```python
from build123d import *

# Parameters (mm, degrees)
F0_R         = 10
F1_DEPTH     = 15
F2_R         = 15
F3_T1_DEPTH  = 32.0168478214
F3_T3_DEPTH  = 19.855092474
F3_T5_DEPTH  = 60.8257569496
F3_T7_DEPTH  = 65
F3_T9_DEPTH  = 54.2875458035
F3_T11_DEPTH = 15
F5_R         = 12
F6_DEPTH     = 12
F7_R         = 11.99999
F8_R         = 4.05
F9_DEPTH     = 27.001


# Not quite as in the source:
# - a fillet or chamfer that OpenCascade refuses, or shapes differently, is made with other operations: its cross-section is extruded or revolved along the edge and cut away or added
# - a fillet or chamfer is up to 0.001 mm smaller than in the source, because OpenCascade refuses the exact size


with BuildPart() as f1:
    # F0 (on Front) → F1 (new body)
    with BuildSketch(Plane.XZ):
        Polygon((-138.9475274131, 122.1416580278), (0, 0), (17.5, -71.8808303125), (45.5, -71.8808303125), (45.5, -56.8808303125), (39.5, -56.8808303125), (35, -62), (27, -62), (27, -12), (35, -12), (35, -20), (41, -20), (41, 0), (0, 53.2575148171), (-112.5385202719, 152.1843666577), align=None)
        with Locations((-67.1597420143, 85.6654484175)):
            Circle(F0_R, mode=Mode.SUBTRACT)
        with Locations((-89.6917734867, 105.4722037734)):
            Circle(F0_R, mode=Mode.SUBTRACT)
        with Locations((-44.6277105419, 65.8586930616)):
            Circle(F0_R, mode=Mode.SUBTRACT)
        with Locations((-22.0956790695, 46.0519377058)):
            Circle(F0_R, mode=Mode.SUBTRACT)
    extrude(amount=F1_DEPTH)

    # F2
    f2_edges = [f1.edges().sort_by_distance(p)[0] for p in [
        (-112.53852, -7.5, 152.184367),
        (-138.947527, -7.5, 122.141658),
    ]]
    fillet(f2_edges, radius=F2_R)

    # F3: fillet of radius 10 on 6 edges, made by hand

    # F3_s2 → F3_t1 (cut)
    with BuildSketch(Plane.XZ.offset(-8.5084239107)):
        with BuildLine():
            ThreePointArc((38.9238894384, 2.6967924145), (40.4667548395, -0.1814830349), (41, -3.4033695643))
            Line((41, -3.4033695643), (41.2, -3.4033695643))
            Line((41.2, -3.4033695643), (41.2, 0.0680673913))
            Line((41.2, 0.0680673913), (39.0823672272, 2.8187956541))
            Line((39.0823672272, 2.8187956541), (38.9238894384, 2.6967924145))
        make_face()
    extrude(amount=F3_T1_DEPTH, mode=Mode.SUBTRACT)

    # F3_s4 → F3_t3 (cut)
    with BuildSketch(Plane.XZ.offset(-2.427546237)):
        with BuildLine():
            ThreePointArc((-0.7293006428, 53.8986056762), (-0.0343212423, 53.2253561798), (0.5923370103, 52.4880904975))
            Line((0.5923370103, 52.4880904975), (0.750814799, 52.6100937371))
            Line((0.750814799, 52.6100937371), (0.1466310486, 53.3949065431))
            Line((0.1466310486, 53.3949065431), (-0.5972556071, 54.0488192193))
            Line((-0.5972556071, 54.0488192193), (-0.7293006428, 53.8986056762))
        make_face()
    extrude(amount=F3_T3_DEPTH, mode=Mode.SUBTRACT)

    # F3_s6 → F3_t5 (cut)
    with BuildSketch(Plane.XZ.offset(-22.9128784748)):
        with BuildLine():
            ThreePointArc((45.5, -66.0459817024), (43.8666002653, -60.5687561273), (39.5, -56.8808303125))
            Line((39.5, -56.8808303125), (39.58, -56.6975272847))
            ThreePointArc((39.58, -56.6975272847), (42.5, -56.6808303125), (45.5, -56.6808303125))
            Line((45.5, -56.6808303125), (45.7, -56.8808303125))
            Line((45.7, -56.8808303125), (45.7, -66.0459817024))
            Line((45.7, -66.0459817024), (45.5, -66.0459817024))
        make_face()
    extrude(amount=F3_T5_DEPTH, mode=Mode.SUBTRACT)

    # F3_s8 → F3_t7 (cut)
    with BuildSketch(Plane.XZ.offset(-25)):
        with BuildLine():
            ThreePointArc((35.5, -71.8808303125), (42.5710678119, -68.9518981244), (45.5, -61.8808303125))
            Line((45.5, -61.8808303125), (45.7, -61.8808303125))
            Line((45.7, -61.8808303125), (45.7, -72.0808303125))
            Line((45.7, -72.0808303125), (35.5, -72.0808303125))
            Line((35.5, -72.0808303125), (35.5, -71.8808303125))
        make_face()
    extrude(amount=F3_T7_DEPTH, mode=Mode.SUBTRACT)

    # F3_s10 → F3_t9 (cut)
    with BuildSketch(Plane.XZ.offset(-19.6437729018)):
        with BuildLine():
            ThreePointArc((15.6413136753, -64.2463208091), (19.1791155574, -69.7438737743), (25.3575091607, -71.8808303125))
            Line((25.3575091607, -71.8808303125), (25.3575091607, -72.0808303125))
            Line((25.3575091607, -72.0808303125), (17.3428498168, -72.0808303125))
            Line((17.3428498168, -72.0808303125), (15.4469897656, -64.2936306191))
            Line((15.4469897656, -64.2936306191), (15.6413136753, -64.2463208091))
        make_face()
    extrude(amount=F3_T9_DEPTH, mode=Mode.SUBTRACT)

    # F3_s12 → F3_t11 (join)
    with BuildSketch(Plane.XZ):
        with BuildLine():
            ThreePointArc((-2.3681074114, 2.0816819918), (-0.4151755765, -0.2512704506), (0.7458362887, -3.0635046691))
            Line((0.7458362887, -3.0635046691), (0.9401601984, -3.0161948591))
            Line((0.9401601984, -3.0161948591), (0.1794071839, 0.1085799033))
            Line((0.1794071839, 0.1085799033), (-2.2360623757, 2.2318955349))
            Line((-2.2360623757, 2.2318955349), (-2.3681074114, 2.0816819918))
        make_face()
    extrude(amount=F3_T11_DEPTH)

    # F5 (on face) → F6 (join)
    with BuildSketch(Plane(origin=(0, 0, 0), x_dir=(-1, 0, 0), z_dir=(0, 1, 0))):
        with Locations((111.3978201201, 124.552878143)):
            Circle(F5_R)
    extrude(amount=F6_DEPTH)

    # F7 (radius 12 in the source; OpenCascade refuses exactly that, so slightly less here)
    f7_edges = [f1.edges().sort_by_distance(p)[0] for p in [
        (-99.39782, 12, 124.552878),
    ]]
    fillet(f7_edges, radius=F7_R)

    # F8 (on face) → F9 (cut, through all)
    with BuildSketch(Plane.XZ.offset(15)):
        with Locations((-111.3978201201, 124.552878143)):
            Circle(F8_R)
    extrude(amount=-F9_DEPTH, mode=Mode.SUBTRACT)


solid = f1.part
```
Could you check a few things on this model? Use its own coordinates, in mm. A direction names the side the tool comes from. Round coordinates to 2 decimals unless told otherwise and drop trailing zeros. Loops run counter-clockwise (first coordinate to the right, second up) from the corner with the lowest first, then second, coordinate; pieces in that order, holes last. Notation, with made-up numbers: (44.5, 17.5) - (71.5, 17.5) arc R30 cw to (71.5, 52.5) - close; hole circle Ø9 at (-34, -18). An arc over 180 degrees is marked (long way). Answer in a Markdown table with one row per item. Add a question column.
(1) If we section it at A-A (x = -83): Please give me the cut outline in (y, z).
(2) If we section it at C-C (y = -9): Please give me the cut outline in (x, z).
(3) For faces 1 (the face through (41, -7, -12)), 2 (the face through (-65.9, -7.4, 57.93)), 3 (the face through (38, -7, -20)), 4 (the face through (37.282, -7.395, -59.405)), which set-ups out of +Z, -Z, +X, -X, +Y, -Y let a thin tool reach every point of the face, with its end or its side?
(4) I'm going to push flat-ended pins straight in: pin 1 (2 mm diameter, centred on y = -4, z = 84, fed in from -X); pin 2 (7.5 mm diameter, centred on y = -8, z = -36.5, fed in from +X); pin 3 (1 mm diameter, centred on y = 0, z = 54.5, fed in from -X); pin 4 (5 mm diameter, centred on x = 37.5, y = -6.5, fed in from -Z). Where does each tip first touch, or does it pass through?
(5) If we section it at D-D (x = 22.5): Please give me the cut outline in (y, z).
(6) I need wall thicknesses on line 1 along Z through (x, y) = (-92, -9.5); line 2 along Z through (x, y) = (-113, 5.75); line 3 along X through (y, z) = (-11.25, 61). Which ranges of each line are inside material? Lowest first, please.
(7) If we mould it in two halves opening along Z, with no side actions, what happens to faces 5 (the face through (31, -7, -12)), 6 (the face through (-125.697, -7.395, 137.216)), 7 (the face through (-38, -15, 54))? For each: pulls with the +Z half, pulls with the -Z half, needs draft (parallel to the pull), parting line crosses it, or undercut.
(8) If we section it at B-B (z = 62.5): Please give me the cut outline in (x, y), plus the area to 3 significant figures.
Model answer:
| question | item | result |
|---|---|---|
| 1 | outline | (-15, 72.96) - (0, 72.96) - (0, 98.04) - (-15, 98.04) - close; (-15, 112.9) - (0, 112.9) - (0, 126.22) - (-15, 126.22) - close |
| 2 | outline | (-129.04, 133.41) arc R15 ccw to (-127.68, 112.24) - (-2.37, 2.08) arc R10 cw to (0.75, -3.06) - (15.64, -64.25) arc R10 ccw to (25.36, -71.88) - (35.5, -71.88) arc R10 ccw to (45.28, -63.96) arc R10 ccw to (39.5, -56.88) - (35, -62) - (27, -62) - (27, -12) - (35, -12) - (35, -20) - (41, -20) - (41, -3.4) arc R10 ccw to (38.92, 2.7) - (0.59, 52.49) arc R10 ccw to (-0.73, 53.9) - (-101.27, 142.28) arc R15 ccw to (-122.44, 140.92) - close; hole circle Ø8.1 at (-111.4, 124.55); hole circle Ø20 at (-89.69, 105.47); hole circle Ø20 at (-67.16, 85.67); hole circle Ø20 at (-44.63, 65.86); hole circle Ø20 at (-22.1, 46.05) |
| 3 | face 1 | +Z, +X, +Y, -Y |
| 3 | face 2 | -Z, -X, +Y, -Y |
| 3 | face 3 | +X, +Y, -Y |
| 3 | face 4 | +Y, -Y |
| 4 | pin 1 | stops at x = -96.7 |
| 4 | pin 2 | stops at x = 27 |
| 4 | pin 3 | stops at x = -62.57 |
| 4 | pin 4 | stops at z = -71.88 |
| 5 | outline | (-15, -71.46) - (0, -71.46) - (0, 24.03) - (-15, 24.03) - close |
| 6 | line 1 | z = 80.87 to 95.74, 115.2 to 134.13 |
| 6 | line 2 | z = 114.14 to 120.83, 128.27 to 134.96 |
| 6 | line 3 | x = -69.39 to -53.37, -35.89 to -8.81 |
| 7 | face 5 | undercut |
| 7 | face 6 | pulls with the +Z half |
| 7 | face 7 | needs draft |
| 8 | outline | (-71.1, -15) - (-54.05, -15) - (-54.05, 0) - (-71.1, 0) - close; (-35.21, -15) - (-10.51, -15) - (-10.51, 0) - (-35.21, 0) - close |
| 8 | area | 626 mm² |
